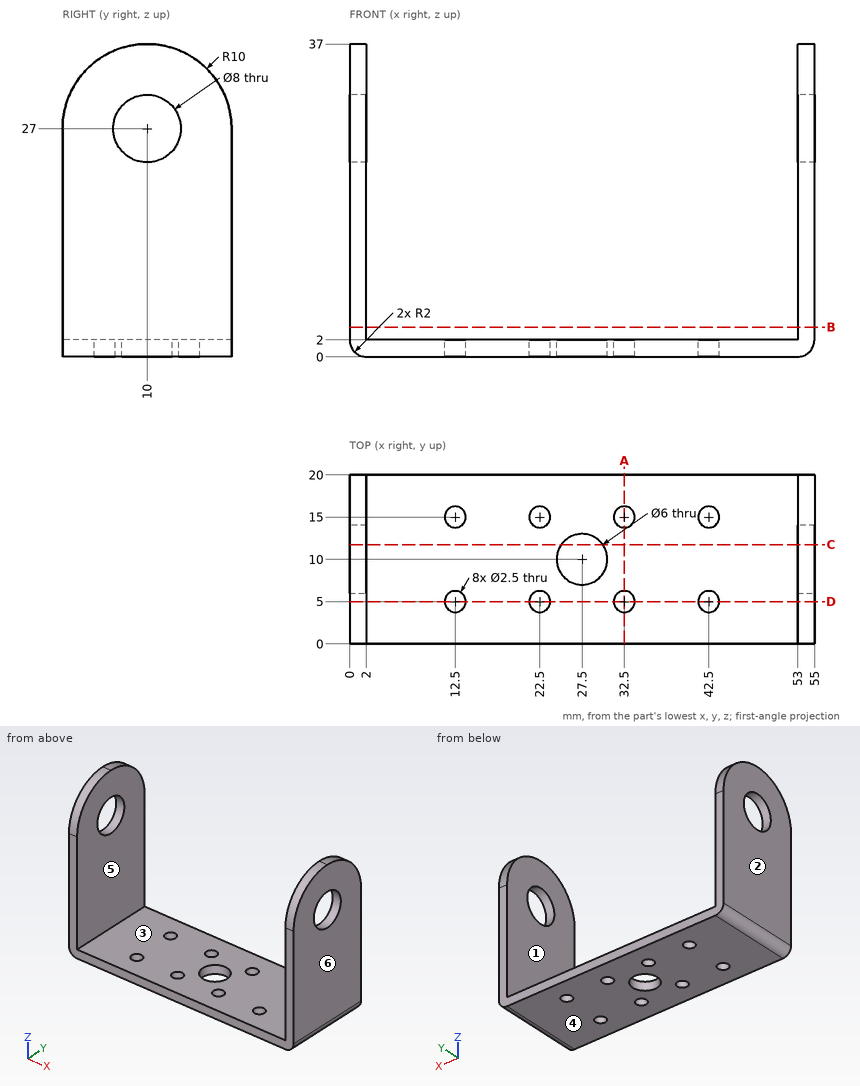
Source: three-view drawing plus pictorial views. Frame: mm from the lowest corner of the part. A direction names the side the tool comes from. Coordinates: 2 decimals unless noted, no trailing zeros. Loops run counter-clockwise (first coordinate to the right, second up) from the corner with the lowest first, then second, coordinate; pieces in that order, holes last. Notation, with made-up numbers: (61.5, -31) -> (65.5, -31) arc R18 ccw to (65.5, -3) -> close; hole circle Ø3 at (-13, 84.25). An arc over 180 degrees is marked (long way). Answer in a Markdown table with one row per item. Add a question column.
Q1. Contact query for flat-ended pins moving along their axis: pin 1 Ø1.5 at (x, y) = (22.5, 5) entering from +Z; pin 2 Ø3 at (x, y) = (42.5, 5) entering from +Z. Output: stop coordinate, or through.
Q2. Section B-B on z = 3.5. Return the cut outline in (x, y), and give its area (3 significant figures).
Q3. Pull-direction query (X, two-part tool) for the marked faces 1, 2, 3 and 4; classes: pulls with the +X half, pulls with the -X half, needs draft (parallel to the pull), parting line crosses it, or undercut.
Q4. Reachability of the marked faces 5 and 6 from +Z, -Z, +X, -X, +Y, -Y: full face, straight path, thin tool, end or side. Return the list, or none.
Q5. Section C-C on y = 11.75. Return the cut outline in (x, z).
Q6. Ray query, line 1 along Y through (x, z) = (42.5, 1.65); line 2 along X through (y, z) = (12.25, 18); line 3 along X through (y, z) = (15, 0.85). Return the intervals inside material, ascending.
Q7. Section D-D on y = 5. Return the cut outline in (x, z), and give its area (3 significant figures).
Q8. Section A-A on x = 32.5. Return the cut outline in (y, z).
Computed values:
| question | item | result |
|---|---|---|
| 1 | pin 1 | passes through |
| 1 | pin 2 | stops at z = 2 |
| 2 | outline | (0, 0) -> (2, 0) -> (2, 20) -> (0, 20) -> close; (53, 0) -> (55, 0) -> (55, 20) -> (53, 20) -> close |
| 2 | area | 80.0 mm^2 |
| 3 | face 1 | undercut |
| 3 | face 2 | pulls with the -X half |
| 3 | face 3 | undercut |
| 3 | face 4 | needs draft |
| 4 | face 5 | +Z, +Y, -Y |
| 4 | face 6 | +Z, -Z, +X, +Y, -Y |
| 5 | outline | (0, 2) arc R2 ccw to (2, 0) -> (25.06, 0) -> (25.06, 2) -> (2, 2) -> (2, 23.4) -> (0, 23.4) -> close; (0, 30.6) -> (2, 30.6) -> (2, 36.85) -> (0, 36.85) -> close; (29.94, 0) -> (53, 0) arc R2 ccw to (55, 2) -> (55, 23.4) -> (53, 23.4) -> (53, 2) -> (29.94, 2) -> close; (53, 30.6) -> (55, 30.6) -> (55, 36.85) -> (53, 36.85) -> close |
| 6 | line 1 | y = 0 to 3.75, 6.25 to 13.75, 16.25 to 20 |
| 6 | line 2 | x = 0 to 2, 53 to 55 |
| 6 | line 3 | x = 0.36 to 11.25, 13.75 to 21.25, 23.75 to 31.25, 33.75 to 41.25, 43.75 to 54.64 |
| 7 | outline | (0, 2) arc R2 ccw to (2, 0) -> (11.25, 0) -> (11.25, 2) -> (2, 2) -> (2, 35.66) -> (0, 35.66) -> close; (13.75, 0) -> (21.25, 0) -> (21.25, 2) -> (13.75, 2) -> close; (23.75, 0) -> (31.25, 0) -> (31.25, 2) -> (23.75, 2) -> close; (33.75, 0) -> (41.25, 0) -> (41.25, 2) -> (33.75, 2) -> close; (43.75, 0) -> (53, 0) arc R2 ccw to (55, 2) -> (55, 35.66) -> (53, 35.66) -> (53, 2) -> (43.75, 2) -> close |
| 7 | area | 223 mm^2 |
| 8 | outline | (0, 0) -> (3.75, 0) -> (3.75, 2) -> (0, 2) -> close; (6.25, 0) -> (13.75, 0) -> (13.75, 2) -> (6.25, 2) -> close; (16.25, 0) -> (20, 0) -> (20, 2) -> (16.25, 2) -> close |
